Build history of the part. All positions in model axes, mm. A direction names the side the tool comes from. Coordinates: 2 decimals unless noted, no trailing zeros. Loops run counter-clockwise (first coordinate to the right, second up) from the corner with the lowest first, then second, coordinate; pieces in that order, holes last.
Item 1: Cut at D-D (y = -8.5). List the corners of the cut face in (x, z) (3 decimals).
Item 2: Cut at A-A (y = -38.1). List the corners of the cut face in (x, z) (3 decimals), and give its area (3 significant figures).
Item 3: Flat gauge pins, fed straight in: pin 1 (2 mm diameter, centred on x = 54, y = -43, fed in from +Z); pin 2 (10 mm diameter, centred on y = -40, z = 88.5, fed in from +X); pin 3 (10 mm diameter, centred on x = 23.5, z = 12.5, fed in from +Y); pin 4 (22.5 mm diameter, centred on y = -39, z = 59, fed in from +X). Where does each tip first touch, or does it go through?
Item 4: 3-axis set-ups, long thin cutter, end or side, ignore diameter. For faces 1 (the face through (38.795, -69.939, 92.164)), 2 (the face through (120, -38, 28.575)), 3 (the face through (157.87, -32.38, 22.31)): which of +Z, -Z, +X, -X, +Y, -Y reach the whole face in a straight line?
Item 5: Mould opens along X. For faces 4 (the face through (148, -38, 15.875)), 5 (the face through (0, -38, 37)), 6 (the face through (177.8, -38, 14)), 7 (the face through (41, -63.5, 69)) say: released by +X, released by -X, zero draft, split by the parting line, or undercut.
Item 6: Drill centre lines: line 1 along Y through (x, z) = (139.7, 25.5); line 2 along Z through (x, y) = (166, -31) (3 decimals); line 3 along X through (y, z) = (-19, 76). Where is each one in solid material? Low to high.
Item 7: Cut at B-B (z = 76.2). List the corners of the cut face in (x, y) (3 decimals), and give its area (3 significant figures).
Item 8: Cut at C-C (x = 139.7). List the corners of the cut face in (y, z) (3 decimals).
from build123d import *

# Parameters (mm, degrees)
F1_DEPTH  = 76.2
F3_DEPTH  = 76.201
F4_R      = 19.05
F5_DEPTH  = 12.7
F6_R      = 6.35
F7_DEPTH  = 76.201
F8_R      = 19.05
F9_DEPTH  = 12.7
F10_R     = 6.35
F11_DEPTH = 114.552047


with BuildPart() as f1:
    # F0 (on Front) → F1 (new body)
    with BuildSketch(Plane.XZ):
        Polygon((0, 127), (0, 0), (177.8, 0), (177.8, 28.575), (82.55, 28.575), (82.55, 127), align=None)
    extrude(amount=F1_DEPTH)

    # F2 (on face) → F3 (cut, through all)
    with BuildSketch(Plane.XZ.offset(76.2)):
        with BuildLine():
            ThreePointArc((0, 73.276047), (41.275, 114.551047), (82.55, 73.276047))
            Line((82.55, 73.276047), (82.55, 127))
            Line((82.55, 127), (0, 127))
            Line((0, 127), (0, 73.276047))
        make_face()
    extrude(amount=-F3_DEPTH, mode=Mode.SUBTRACT)

    # F4 (on face) → F5 (cut)
    with BuildSketch(Plane.XZ.offset(76.2)):
        with Locations((41.275, 73.276047)):
            Circle(F4_R)
    extrude(amount=-F5_DEPTH, mode=Mode.SUBTRACT)

    # F6 (on face) → F7 (cut, through all)
    with BuildSketch(Plane(origin=(0, 0, 0), x_dir=(-1, 0, 0), z_dir=(0, 1, 0))):
        with Locations((-41.275, 76.2)):
            Circle(F6_R)
    extrude(amount=-F7_DEPTH, mode=Mode.SUBTRACT)

    # F8 (on face) → F9 (cut)
    with BuildSketch(Plane.XY.offset(28.575)):
        with Locations((139.7, -38.1)):
            Circle(F8_R)
    extrude(amount=-F9_DEPTH, mode=Mode.SUBTRACT)

    # F10 (on face) → F11 (cut, through all)
    with BuildSketch(Plane(origin=(0, 0, 0), x_dir=(1, 0, 0), z_dir=(0, 0, -1))):
        with Locations((139.7, 38.1)):
            Circle(F10_R)
    extrude(amount=-F11_DEPTH, mode=Mode.SUBTRACT)


solid = f1.part
Filled sheet:
1. outline: (0, 0) - (177.8, 0) - (177.8, 28.575) - (82.55, 28.575) - (82.55, 73.276) arc R41.275 ccw to (0, 73.276) - close; hole circle Ø12.7 at (41.275, 76.2)
2. outline: (0, 0) - (133.35, 0) - (133.35, 15.875) - (120.65, 15.875) - (120.65, 28.575) - (82.55, 28.575) - (82.55, 73.276) arc R41.275 ccw to (0, 73.276) - close; (146.05, 0) - (177.8, 0) - (177.8, 28.575) - (158.75, 28.575) - (158.75, 15.875) - (146.05, 15.875) - close; hole circle Ø12.7 at (41.275, 76.2)
2. area: 10,600 mm2
3. pin 1: stops at z = 112.85
3. pin 2: stops at x = 81.26
3. pin 3: stops at y = 0
3. pin 4: stops at x = 82.55
4. face 1: -Y
4. face 2: +Z, +X, +Y, -Y
4. face 3: +Z
5. face 4: undercut
5. face 5: released by -X
5. face 6: released by +X
5. face 7: undercut
6. line 1: y = -76.2 to -57.15, -19.05 to 0
6. line 2: z = 0 to 28.575
6. line 3: x = 0.09 to 34.93, 47.62 to 82.46
7. outline: (0.104, -76.2) - (22.451, -76.2) - (22.451, -63.5) - (34.925, -63.5) - (34.925, 0) - (0.104, 0) - close; (47.625, -63.5) - (60.099, -63.5) - (60.099, -76.2) - (82.446, -76.2) - (82.446, 0) - (47.625, 0) - close
7. area: 4,990 mm2
8. outline: (-76.2, 0) - (-44.45, 0) - (-44.45, 15.875) - (-57.15, 15.875) - (-57.15, 28.575) - (-76.2, 28.575) - close; (-31.75, 0) - (0, 0) - (0, 28.575) - (-19.05, 28.575) - (-19.05, 15.875) - (-31.75, 15.875) - close
